For this review, take the finished solid that the model builds, in its own axes (mm). Face numbers are marked on the shaded views. A direction names the side the tool comes from. Round coordinates to 2 decimals unless told otherwise and drop trailing zeros. Loops run counter-clockwise (first coordinate to the right, second up) from the corner with the lowest first, then second, coordinate; pieces in that order, holes last. Notation, with made-up numbers: (-1, 7) -> (48, 7) arc R8 cw to (48, 19) -> close; hole circle Ø2 at (49, 42). An arc over 180 degrees is marked (long way). One line per question, with ' | ' between items. Start each with the question number.
1. For the marked faces 1, 2 and 3, list the 3-axis set-ups (+Z, -Z, +X, -X, +Y, -Y) from which the entire face can be reached by the end or side of a thin tool; tool diameter is ignored.
2. Consider section B-B (z = 35). Write out the cut boundary in (x, y).
3. Consider section A-A (z = 2.5). Write out the cut boundary in (x, y), and give its area (3 significant figures).
4. Consider section C-C (y = 25). Write out the cut boundary in (x, z).
5. Consider section D-D (z = 15). Write out the cut boundary in (x, y), and give its area (3 significant figures).
6. For pin 1 Ø2.5 at (x, y) = (12, 13) entering from -Z; pin 2 Ø10 at (y, z) = (34, 15.5) entering from +X; pin 3 Ø4.5 at (x, y) = (11.5, 16) entering from -Z, all flat-tipped, find the tip position at first contact; note any pin that passes through.
7. Wall thickness on line 1 along Y through (x, z) = (12, 3.25); line 2 along Z through (x, y) = (12.5, 2.6); line 3 along Y through (x, z) = (14, 9): over which ranges is each line inside the solid? List them lowest first.
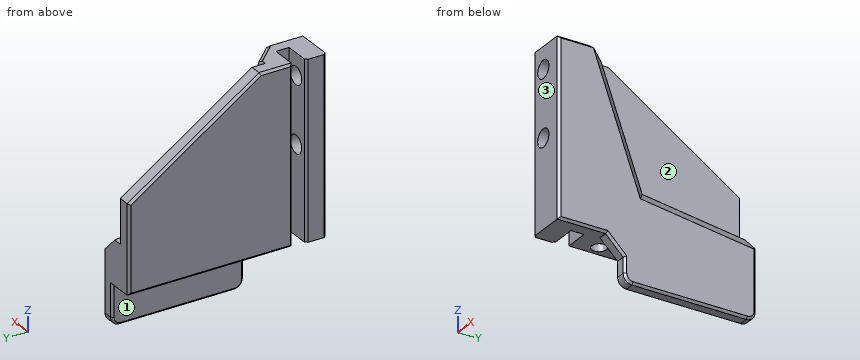
```python
from build123d import *
from OCP.BRepFilletAPI import BRepFilletAPI_MakeChamfer

# Parameters (mm, degrees)
SKETCH1_W           = 9
SKETCH1_H           = 45
SKETCH1_R           = 1.63195
BOSS_EXTRUDE1_DEPTH = 40
SKETCH1_3_R         = 1.63195
CUT_EXTRUDE1_DEPTH  = 10
SKETCH2_W           = 40
SKETCH2_H           = 3
CUT_EXTRUDE2_DEPTH  = 6
CUT_EXTRUDE3_DEPTH  = 9
CUT_EXTRUDE4_DEPTH  = 6
CHAMFER2_SIZE       = 4
SKETCH6_R           = 2.0193
CUT_EXTRUDE5_DEPTH  = 6
SKETCH7_W           = 3
SKETCH7_H           = 30
BOSS_EXTRUDE3_DEPTH = 9.52
CHAMFER3_SIZE       = 4
FILLET1_R           = 2
CHAMFER4_SIZE       = 0.5
CHAMFER4_SIZE2      = 0.681231536
SKETCH8_W           = 73.765636672
SKETCH8_H           = 62.769253432
CUT_EXTRUDE6_DEPTH  = 9


with BuildPart() as part:
    # Sketch1 → Boss-Extrude1 (new body)
    # profile 1 of 3: a face of its own
    with BuildSketch(Plane.XY):
        with Locations((4.5, 22.5)):
            Rectangle(SKETCH1_W, SKETCH1_H)
        with Locations((6, 13)):
            Circle(SKETCH1_R, mode=Mode.SUBTRACT)
        with Locations((6, 25)):
            Circle(SKETCH1_R, mode=Mode.SUBTRACT)
    # profile 2 of 3: a face of its own
    with BuildSketch(Plane.XY):
        with Locations((6, 25)):
            Circle(SKETCH1_R)
    # profile 3 of 3: a face of its own
    with BuildSketch(Plane.XY):
        with Locations((6, 13)):
            Circle(SKETCH1_R)
    extrude(amount=BOSS_EXTRUDE1_DEPTH)

    # Sketch1<3> → Cut-Extrude1 (cut)
    with BuildSketch(Plane.XY):
        with Locations((6, 25)):
            Circle(SKETCH1_3_R)
        with Locations((6, 13)):
            Circle(SKETCH1_3_R)
    extrude(amount=CUT_EXTRUDE1_DEPTH, mode=Mode.SUBTRACT)

    # Sketch2 → Cut-Extrude2 (cut)
    with BuildSketch(Plane(origin=(9, 0, 0), x_dir=(0, 0, -1), z_dir=(1, 0, 0))):
        with Locations((-20, 6.2)):
            Rectangle(SKETCH2_W, SKETCH2_H)
    extrude(amount=-CUT_EXTRUDE2_DEPTH, mode=Mode.SUBTRACT)

    # Sketch3 → Cut-Extrude3 (cut)
    with BuildSketch(Plane(origin=(9, 0, 0), x_dir=(0, 0, -1), z_dir=(1, 0, 0))):
        Polygon((-20, 45), (-40, 15), (-48.379363257, 51.913157268), align=None)
    extrude(amount=-CUT_EXTRUDE3_DEPTH, mode=Mode.SUBTRACT)

    # Sketch5 → Cut-Extrude4 (cut)
    with BuildSketch(Plane.ZY):
        Polygon((20, 45), (10, 45), (13.204776383, 21.55213026), (40, 12), (40, 15), align=None)
    extrude(amount=-CUT_EXTRUDE4_DEPTH, mode=Mode.SUBTRACT)

    # Chamfer2
    chamfer2_edges = [part.edges().sort_by_distance(p)[0] for p in [
        (0, 33.27606513, 11.602388192),
        (0, 16.77606513, 26.602388192),
    ]]
    chamfer(chamfer2_edges, length=CHAMFER2_SIZE)

    # Sketch6 → Cut-Extrude5 (cut)
    with BuildSketch(Plane.XZ):
        with Locations(Location((5.5, 35, 0), (0, 0, 270))):
            Circle(SKETCH6_R)
        with Locations(Location((5.5, 20, 0), (0, 0, 270))):
            Circle(SKETCH6_R)
    extrude(amount=-CUT_EXTRUDE5_DEPTH, mode=Mode.SUBTRACT)

    # Sketch7 → Boss-Extrude3 (add)
    with BuildSketch(Plane(origin=(0, 0, 0), x_dir=(-1, 0, 0), z_dir=(0, 0, -1))):
        with Locations((-1.5, 30)):
            Rectangle(SKETCH7_W, SKETCH7_H)
    extrude(amount=BOSS_EXTRUDE3_DEPTH)

    # Chamfer3
    chamfer3_edges = [part.edges().sort_by_distance(p)[0] for p in [
        (1.5, 15, 0),
    ]]
    chamfer(chamfer3_edges, length=CHAMFER3_SIZE)

    # Fillet1
    fillet1_edges = [part.edges().sort_by_distance(p)[0] for p in [
        (1.5, 45, -9.52),
        (1.5, 15, -9.52),
    ]]
    fillet(fillet1_edges, radius=FILLET1_R)

    # Chamfer4: one chamfer whose edges measure the first distance from different faces: ONE call of the kernel's chamfer builder (chamfer() names one face for all edges)
    chamfer4_edges_1 = [part.edges().sort_by_distance(p)[0] for p in [
        (3, 45, -3.76),
        (3, 44.414213562, -8.934213562),
        (3, 15, -5.76),
        (3, 30, -9.52),
        (3, 15.585786438, -8.934213562),
        (3, 13, -2),
        (9, 7.7, 20),
        (9, 4.7, 20),
        (0, 3.876717178, 40),
        (0, 0, 20),
        (0, 5.5, 0),
        (0, 13, -2),
        (0, 15, -5.76),
        (0, 45, -0.778594073),
        (0, 15.585786438, -8.934213562),
        (0, 44.414213562, -8.934213562),
        (0, 30, -9.52),
        (9, 0, 20),
        (9, 11.35, 40),
        (9, 30, 30),
        (9, 45, 10),
        (9, 26.35, 0),
    ]]
    chamfer4_edges_2 = [part.edges().sort_by_distance(p)[0] for p in [
        (2, 9.876717178, 40),
    ]]
    chamfer4_side_2 = [part.faces().sort_by_distance(p)[0] for p in [
        (1.957665589, 14.938546455, 25.674700071),
    ]]
    chamfer4 = BRepFilletAPI_MakeChamfer(part.part.solid().wrapped)
    for e in chamfer4_edges_1:
        chamfer4.Add(CHAMFER4_SIZE, e.wrapped)
    for e in chamfer4_edges_2:
        chamfer4.Add(CHAMFER4_SIZE, CHAMFER4_SIZE2, e.wrapped, chamfer4_side_2[0].wrapped)  # the first distance lies on this face
    add(Compound.cast(chamfer4.Shape()), mode=Mode.REPLACE)

    # Mirror1: part across plane


with BuildPart() as part_1:
    add(part.part)
    add(part.part.mirror(Plane(origin=(9, 0, 40), x_dir=(0, 0, 1), z_dir=(-1, 0, 0))))

    # Sketch8 → Cut-Extrude6 (cut)
    with BuildSketch(Plane.ZY):
        with Locations((15.385718854, 24.547909709)):
            Rectangle(SKETCH8_W, SKETCH8_H)
    extrude(amount=-CUT_EXTRUDE6_DEPTH, mode=Mode.SUBTRACT)


solid = part_1.part
```
Answer block:
1) face 1: -Z, -X, +Y, -Y | face 2: +Z, +X, +Y | face 3: +Z, -Z, +X, -X, -Y
2) outline: (9, 0.5) -> (9.5, 0) -> (10.48, 0) -> (10.48, 4.7) -> (9.5, 4.7) -> (9, 4.2) -> close; (9, 8.2) -> (9.5, 7.7) -> (15, 7.7) -> (15, 4.7) -> (14.52, 4.7) -> (14.52, 0) -> (17.5, 0) -> (18, 0.5) -> (18, 9.54) -> (14, 13.78) -> (12, 13.78) -> (12, 22.5) -> (9.5, 22.5) -> (9, 21.6) -> close
3) outline: (9, 0.5) -> (9.5, 0) -> (17.5, 0) -> (18, 0.5) -> (18, 44.5) -> (17.5, 45) -> (9.5, 45) -> (9, 44.5) -> (9, 8.2) -> (9.5, 7.7) -> (15, 7.7) -> (15, 4.7) -> (9.5, 4.7) -> (9, 4.2) -> close; hole circle Ø3.26 at (12, 13); hole circle Ø3.26 at (12, 25) | area: 370 mm2
4) outline: (9, 0.5) -> (9.5, 0) -> (10.37, 0) -> (10.37, 10) -> (13.63, 10) -> (13.63, 0) -> (15, 0) -> (15, -9.02) -> (15.5, -9.52) -> (17.5, -9.52) -> (18, -9.02) -> (18, 8.7) -> (14, 12.73) -> (12, 12.73) -> (12, 33.33) -> (9.5, 33.33) -> (9, 32.73) -> close
5) outline: (9, 0.5) -> (9.5, 0) -> (17.5, 0) -> (18, 0.5) -> (18, 16.67) -> (14, 20.91) -> (12, 20.91) -> (12, 45) -> (9.5, 45) -> (9, 44.5) -> (9, 8.2) -> (9.5, 7.7) -> (15, 7.7) -> (15, 4.7) -> (9.5, 4.7) -> (9, 4.2) -> close | area: 233 mm2
6) pin 1: stops at z = 10 | pin 2: stops at x = 15.04 | pin 3: stops at z = 0
7) line 1: y = 0 to 4.7, 7.7 to 11.37, 14.63 to 23.37, 26.63 to 45 | line 2: z = 0 to 17.98, 22.02 to 32.98, 37.02 to 40 | line 3: y = 0 to 4.7, 7.7 to 45
